Here's how the part is built. I have some questions about the finished solid (model axes, mm). Face numbers are marked on the shaded views. Round coordinates to 2 decimals unless told otherwise and drop trailing zeros. Order: outer loops, then holes, each group sorted by start corner. A loop starts at its lowest first (then second) coordinate and runs counter-clockwise, first axis right, second up. Notation, with made-up numbers: (-14.75, 65) - (20.25, 65) arc R19 cw to (20.25, 78) - close; hole circle Ø6 at (84.25, 37). An arc over 180 degrees is marked (long way). One line per item, written item: value.
from build123d import *

# Parameters (mm, degrees)
ESQUISSE1_W             = 50
ESQUISSE1_H             = 450
BOSS_EXTRU_1_DEPTH      = 20
ENL_V_MAT_EXTRU_1_REACH = 229.266
ESQUISSE2_R             = 10
CONG_1_R                = 25


with BuildPart() as part:
    # Esquisse1 → Boss.-Extru.1 (new body)
    with BuildSketch(Plane.XY):
        Rectangle(ESQUISSE1_W, ESQUISSE1_H)
    extrude(amount=BOSS_EXTRU_1_DEPTH)

    # Esquisse2 → Enlèv. mat.-Extru.1 (cut, up to next)
    with BuildSketch(Plane.XY.offset(20), mode=Mode.PRIVATE) as enl_v_mat_extru_1_sk1:
        with Locations((0, -200)):
            Circle(ESQUISSE2_R)
    enl_v_mat_extru_1_tool1 = extrude(enl_v_mat_extru_1_sk1.sketch, amount=-ENL_V_MAT_EXTRU_1_REACH, mode=Mode.PRIVATE) & part.part
    # Esquisse2 → Enlèv. mat.-Extru.1 (cut, up to next)
    with BuildSketch(Plane.XY.offset(20), mode=Mode.PRIVATE) as enl_v_mat_extru_1_sk2:
        with Locations((0, 200)):
            Circle(ESQUISSE2_R)
    enl_v_mat_extru_1_tool2 = extrude(enl_v_mat_extru_1_sk2.sketch, amount=-ENL_V_MAT_EXTRU_1_REACH, mode=Mode.PRIVATE) & part.part
    # Esquisse2 → Enlèv. mat.-Extru.1 (cut, up to next)
    with BuildSketch(Plane.XY.offset(20), mode=Mode.PRIVATE) as enl_v_mat_extru_1_sk3:
        Circle(ESQUISSE2_R)
    enl_v_mat_extru_1_tool3 = extrude(enl_v_mat_extru_1_sk3.sketch, amount=-ENL_V_MAT_EXTRU_1_REACH, mode=Mode.PRIVATE) & part.part
    add(enl_v_mat_extru_1_tool1.solids().sort_by_distance((0, -200, 20))[0], mode=Mode.SUBTRACT)
    add(enl_v_mat_extru_1_tool2.solids().sort_by_distance((0, 200, 20))[0], mode=Mode.SUBTRACT)
    add(enl_v_mat_extru_1_tool3.solids().sort_by_distance((0, 0, 20))[0], mode=Mode.SUBTRACT)

    # Congé1
    cong_1_edges = [part.edges().sort_by_distance(p)[0] for p in [
        (-25, -225, 10),
        (25, -225, 10),
        (-25, 225, 10),
        (25, 225, 10),
    ]]
    fillet(cong_1_edges, radius=CONG_1_R - 0.0001)  # a hair under: the kernel refuses the full size


solid = part.part
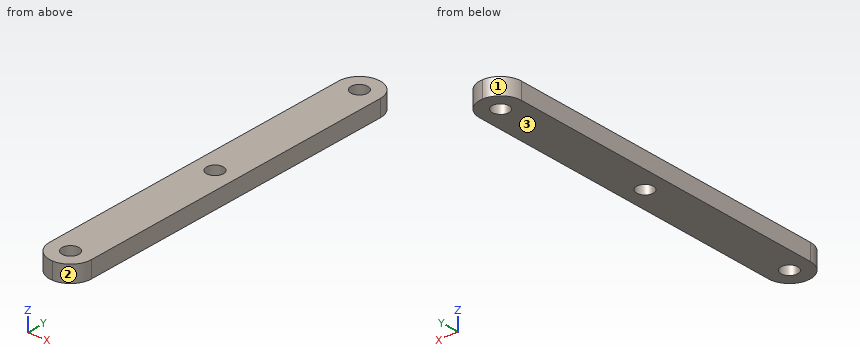
Q1. If I drill on line 1 along Y through (x, z) = (0, 7.5); line 2 along Y through (x, z) = (-10.5, 19); line 3 along Y through (x, z) = (20, 6), over which ranges is the centre line in solid material (lowest first)?
Results list:
line 1: -225 to -210, -190 to -10, 10 to 190, 210 to 225
line 2: -222.69 to 222.69
line 3: -215 to 215
Q2. If we section it at A-A, the plane z = 13: Give the number of separate pieces and of enclosed holes in the cut face, then the cut area to 3 significant figures.
Results list:
separate pieces: 1
enclosed holes: 3
area: 21,000 mm²
Q3. Will these pins go through, and if not, where does the flat tip stop? pin 1 (10 mm diameter, centred on x = -19, z = 10, fed in from +Y); pin 2 (1.5 mm diameter, centred on x = 3.5, z = 9, fed in from +Y); pin 3 (2 mm diameter, centred on x = 15.5, z = 7.5, fed in from +Y).
Results list:
pin 1: y = 220.71
pin 2: y = 224.85
pin 3: y = 220.37
Q4. If we section it at B-B, the plane y = 0: Please give me the cut outline in (x, z).
Results list:
outline: (-25, 0) - (-10, 0) - (-10, 20) - (-25, 20) - close; (10, 0) - (25, 0) - (25, 20) - (10, 20) - close
Q5. If we section it at C-C, the plane y = 194: Please give me the cut outline in (x, z), then the cut area to 3 significant figures.
Results list:
outline: (-25, 0) - (-8, 0) - (-8, 20) - (-25, 20) - close; (8, 0) - (25, 0) - (25, 20) - (8, 20) - close
area: 680 mm²
Q6. If we section it at D-D, the plane x = 18.5: Please give me the cut outline in (y, z).
Results list:
outline: (-216.82, 0) - (216.82, 0) - (216.82, 20) - (-216.82, 20) - close
Q7. We'd pull the mould along X, two halves only. Please class the marked faces 1, 2 and 3: released by +X, released by -X, zero draft, split by the parting line, or undercut.
Results list:
face 1: released by -X
face 2: released by +X
face 3: zero draft
